```python
from build123d import *

# Parameters (mm, degrees)
BOSS_EXTRUDE1_DEPTH = 5
BOSS_EXTRUDE2_DEPTH = 15
CUT_EXTRUDE1_REACH  = 56.699
SKETCH3_R           = 4.1
CUT_EXTRUDE2_DEPTH  = 6.4
SKETCH9_W           = 13
SKETCH9_H           = 18
CUT_EXTRUDE3_DEPTH  = 55.699177325


# Read off the part's stored shape, not the designer's step: Boss-Extrude2
with BuildPart() as part:
    # Sketch1 → Boss-Extrude1 (new body)
    with BuildSketch(Plane(origin=(0, 0, 0), x_dir=(1, 0, 0), z_dir=(0, 1, 0))):
        with BuildLine():
            Line((35.986108431, -1), (12.560254774, -1))
            ThreePointArc((12.560254774, -1), (-12.6, 0), (12.560254774, 1))
            Line((12.560254774, 1), (35.986108431, 1))
            ThreePointArc((35.986108431, 1), (-36, 0), (35.986108431, -1))
        make_face()
    extrude(amount=BOSS_EXTRUDE1_DEPTH)

    # Boss-Extrude2 outline → Boss-Extrude2 (add)
    with BuildSketch(Plane(origin=(0, 5, 0), x_dir=(1, 0, 0), z_dir=(0, 1, 0))):
        with BuildLine():
            Line((33.084890811, -1), (12.560254774, -1))
            ThreePointArc((12.560254774, -1), (-12.6, 0), (12.560254774, 1))
            Line((12.560254774, 1), (33.084890811, 1))
            ThreePointArc((33.084890811, 1), (-33.1, 0), (33.084890811, -1))
        make_face()
    extrude(amount=BOSS_EXTRUDE2_DEPTH)

    # Sketch3 → Cut-Extrude1 (cut, up to next)
    with BuildSketch(Plane.XZ, mode=Mode.PRIVATE) as cut_extrude1_sk1:
        with Locations(Location((0, 25, 0), (0, 0, 270))):
            Circle(SKETCH3_R)
    cut_extrude1_tool1 = extrude(cut_extrude1_sk1.sketch, amount=-CUT_EXTRUDE1_REACH, mode=Mode.PRIVATE) & part.part
    # Sketch3 → Cut-Extrude1 (cut, up to next)
    with BuildSketch(Plane.XZ, mode=Mode.PRIVATE) as cut_extrude1_sk2:
        with Locations(Location((0, -25, 0), (0, 0, 270))):
            Circle(SKETCH3_R)
    cut_extrude1_tool2 = extrude(cut_extrude1_sk2.sketch, amount=-CUT_EXTRUDE1_REACH, mode=Mode.PRIVATE) & part.part
    add(cut_extrude1_tool1.solids().sort_by_distance((0, 0, 25))[0], mode=Mode.SUBTRACT)
    add(cut_extrude1_tool2.solids().sort_by_distance((0, 0, -25))[0], mode=Mode.SUBTRACT)

    # Sketch8 → Cut-Extrude2 (cut)
    with BuildSketch(Plane.XZ):
        Polygon((6.618426782, 21.22158407), (6.581417572, 28.842517761), (-0.03700921, 32.620933691), (-6.618426782, 28.77841593), (-6.581417572, 21.157482239), (0.03700921, 17.379066309), align=None)
        Polygon((6.618426782, -28.77841593), (6.581417572, -21.157482239), (-0.03700921, -17.379066309), (-6.618426782, -21.22158407), (-6.581417572, -28.842517761), (0.03700921, -32.620933691), align=None)
    extrude(amount=-CUT_EXTRUDE2_DEPTH, mode=Mode.SUBTRACT)

    # Sketch9 → Cut-Extrude3 (cut, through all)
    with BuildSketch(Plane(origin=(0, 20, 0), x_dir=(1, 0, 0), z_dir=(0, 1, 0))):
        with Locations((-40, 0)):
            Rectangle(SKETCH9_W, SKETCH9_H)
    extrude(amount=-CUT_EXTRUDE3_DEPTH, mode=Mode.SUBTRACT)


solid = part.part
```
For this review, take the finished solid that the model builds, in its own axes (mm). A direction names the side the tool comes from. Give positions to 0.01 mm unless a question says otherwise; leave off trailing zeros. Order: outer loops, then holes, each group sorted by start corner. A loop starts at its lowest first (then second) coordinate and runs counter-clockwise, first axis right, second up.
1) Insertion check: pin 1 (9.5 mm diameter, centred on x = 0, z = -25, fed in from -Y); pin 2 (1.5 mm diameter, centred on x = -34, y = 3.5, fed in from +Z); pin 3 (1 mm diameter, centred on x = 25, y = 6.5, fed in from -Z). Each pin has a flat end and moves straight along its axis. Give the tip position at first contact, or say it passes through.
2) Take a section at C-C (z = 25). Give the boundary of the cut face in (x, y).
3) Take a section at A-A (y = 13.75). Give the boundary of the cut face in (x, z), then the cut area to 3 significant figures.
4) The part is to be moulded in two halves that separate along Z. For faces 1 (the face through (-33.07, 12.4, -1.44)), 2 (the face through (0, 20, 14)), 3 (the face through (24, 10, -1)), 4 (the face through (-33.5, 3, 0)), say which applies: released by +Z, released by -Z, zero draft, split by the parting line, or undercut.
5) Wall thickness on line 1 (X direction, y = 14.75, z = -25); line 2 (X direction, y = 9, z = -10); line 3 (X direction, y = 4.75, z = 0): over which ranges is each line inside the solid? List them lowest first.
6) For faces 5 (the face through (29.3, 5, -16.2)), 6 (the face through (24, 10, 1)), 7 (the face through (3.319, 3.155, 30.705)), 8 (the face through (-12.59, 9.86, 0.54)), list the 3-axis set-ups (+Z, -Z, +X, -X, +Y, -Y) from which the entire face can be reached by the end or side of a thin tool; tool diameter is ignored.
7) Take a section at B-B (x = 9). Give the boundary of the cut face in (y, z).
8) Take a section at D-D (z = 0). Give the boundary of the cut face in (x, y).
Derived:
1. pin 1: stops at y = 6.4
1. pin 2: stops at z = 13.8
1. pin 3: stops at z = -22.26
2. outline: (-25.9, 0) - (-6.6, 0) - (-6.6, 6.4) - (-4.1, 6.4) - (-4.1, 20) - (-21.69, 20) - (-21.69, 5) - (-25.9, 5) - close; (4.1, 6.4) - (6.6, 6.4) - (6.6, 0) - (25.9, 0) - (25.9, 5) - (21.69, 5) - (21.69, 20) - (4.1, 20) - close
3. outline: (12.56, -1) arc R12.6 cw (long way) to (12.56, 1) - (33.08, 1) arc R33.1 ccw (long way) to (33.08, -1) - close; hole circle Ø8.2 at (0, -25); hole circle Ø8.2 at (0, 25)
3. area: 2,800 mm2
4. face 1: split by the parting line
4. face 2: zero draft
4. face 3: undercut
4. face 4: undercut
5. line 1: x = -21.69 to -4.1, 4.1 to 21.69
5. line 2: x = -31.55 to -7.67, 7.67 to 31.55
5. line 3: x = -33.5 to -12.6
6. face 5: +Y
6. face 6: +X, +Y, -Y
6. face 7: -Y
6. face 8: +Y, -Y
7. outline: (0, -34.86) - (5, -34.86) - (5, -31.85) - (20, -31.85) - (20, -8.82) - (0, -8.82) - close; (0, 8.82) - (20, 8.82) - (20, 31.85) - (5, 31.85) - (5, 34.86) - (0, 34.86) - close
8. outline: (-33.5, 0) - (-12.6, 0) - (-12.6, 20) - (-33.1, 20) - (-33.1, 5) - (-33.5, 5) - close
